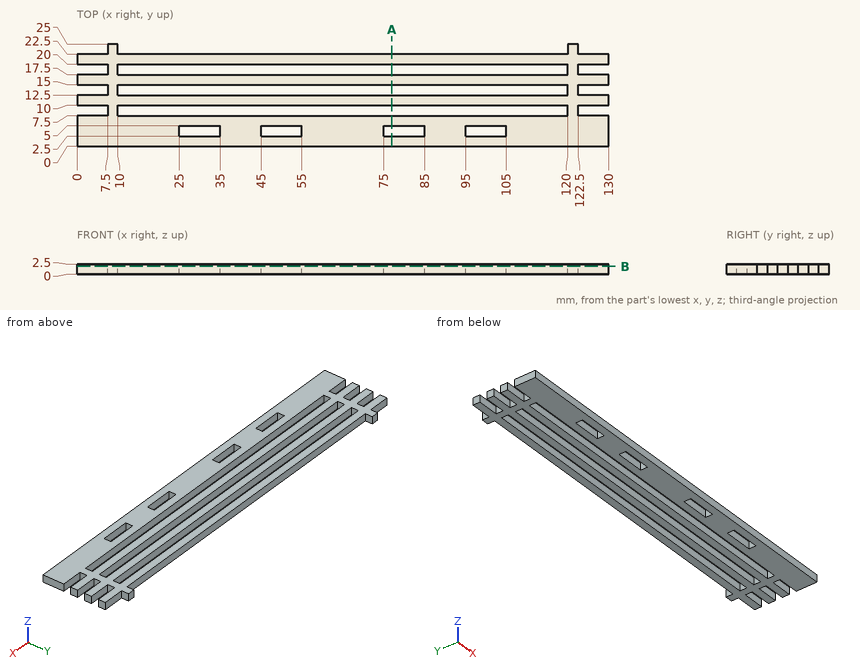
Job drawing, mm, ordinate dimensions from the low corner. One solid piece. Give positions to 0.01 mm unless a question says otherwise; leave off trailing zeros. Loops run counter-clockwise (first coordinate to the right, second up) from the corner with the lowest first, then second, coordinate; pieces in that order, holes last. Notation, with made-up numbers: M 27,47.5 L 41,47.5 A24 ccw 41,79.5 Z; hole C 1,11 d9. An arc over 180 degrees is marked long. Return JSON: item names as keys, results as strings.
1) Flat gauge pins, fed straight in: pin 1 Ø0.8 at (x, z) = (128, 1.5) entering from -Y; pin 2 Ø0.8 at (x, z) = (124.5, 1) entering from +Y; pin 3 Ø0.8 at (y, z) = (19, 1) entering from -X; pin 4 Ø0.8 at (y, z) = (23.5, 0.5) entering from +X. Where does each tip first touch, or does it go through?
Calculated:
{"pin 1": "stops at y = 0", "pin 2": "stops at y = 22.5", "pin 3": "stops at x = 7.5", "pin 4": "stops at x = 122.5"}
2) Saw through at A-A, the plane x = 77. List the corners of the cut face in (y, z).
Calculated:
{"outline": "M 0,0 L 2.5,0 L 2.5,2.5 L 0,2.5 Z; M 5,0 L 7.5,0 L 7.5,2.5 L 5,2.5 Z; M 10,0 L 12.5,0 L 12.5,2.5 L 10,2.5 Z; M 15,0 L 17.5,0 L 17.5,2.5 L 15,2.5 Z; M 20,0 L 22.5,0 L 22.5,2.5 L 20,2.5 Z"}
3) Saw through at B-B, the plane z = 2. Count the separate pieces of the cut face and the enclosed holes in it, then the cut area to 3 significant figures.
Calculated:
{"separate pieces": "1", "enclosed holes": "7", "area": "1,900 mm2"}
4) Drill centre lines: line 1 (Y direction, x = 123.5, z = 0.6); line 2 (Y direction, x = 81.5, z = 1.8); line 3 (X direction, y = 12.75, z = 2). Where is each one in solid material? Low to high.
Calculated:
{"line 1": "y = 0 to 7.5, 10 to 12.5, 15 to 17.5, 20 to 22.5", "line 2": "y = 0 to 2.5, 5 to 7.5, 10 to 12.5, 15 to 17.5, 20 to 22.5", "line 3": "x = 7.5 to 10, 120 to 122.5"}
